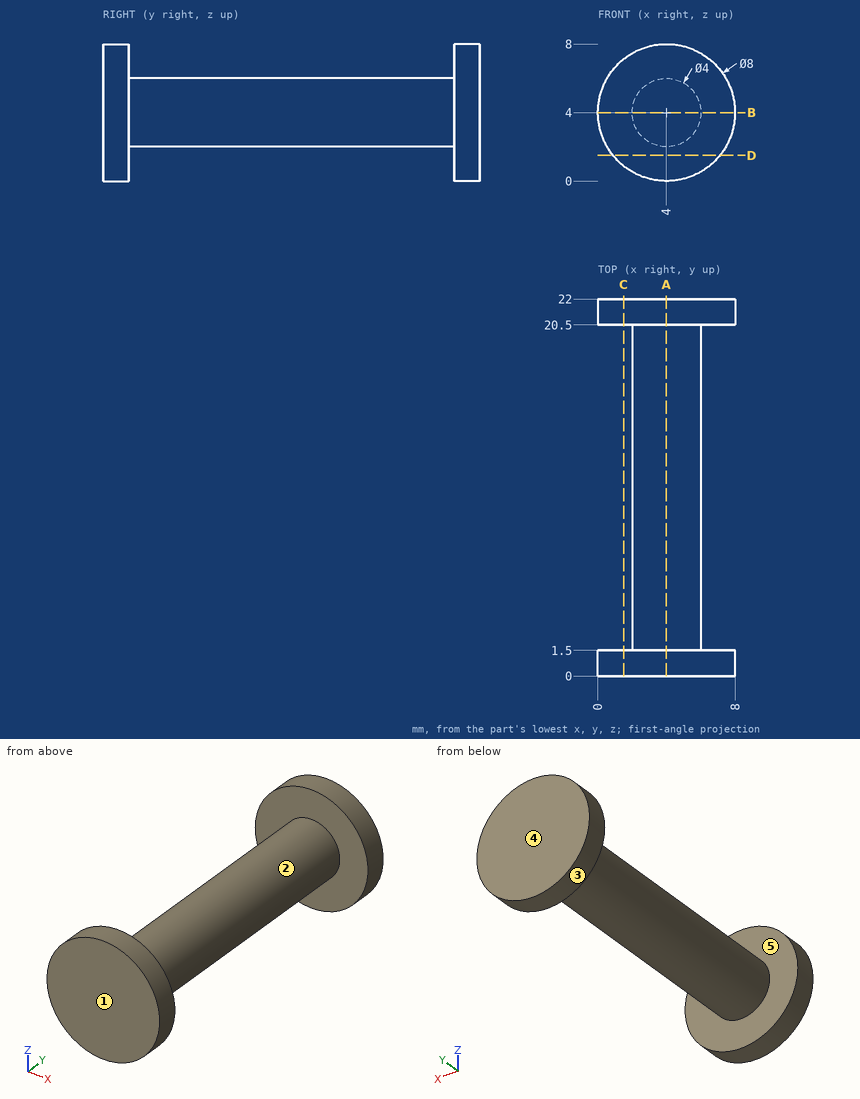
Check sheet for the drawn part. Datum: minimum x, y, z corner. Units: mm. A direction names the side the tool comes from. Round coordinates to 2 decimals unless told otherwise and drop trailing zeros. Write each loop counter-clockwise with the first axis right and the second up, starting at its lowest first coordinate (ties: lowest second). Pieces come first, ordered by that corner, then holes. Notation, with made-up numbers: (-34.75, 11) - (-9.75, 11) arc R27 ccw to (-9.75, 42) - close; hole circle Ø11 at (75, -3.75). An arc over 180 degrees is marked (long way). Return JSON: item names as keys, results as strings.
Q1. Access from +Z, -Z, +X, -X, +Y, -Y to the whole of each face (thin tool, end or side, straight path). Record for the marked faces 4 and 5.
Returned:
{"face 4": "+Z, -Z, +X, -X, +Y", "face 5": "none"}
Q2. Depth check by flat-ended pin: P1, Ø4, axis at y = 10, z = 6, coming from the -X side; P2, Ø1.5, axis at x = 1, y = 19.5, coming from the -Z side; P3, Ø4, axis at x = 6.5, y = 14.5, coming from the +Z side. Enter the tip coordinate at first touch or a pass-through.
Returned:
{"P1": "stops at x = 2", "P2": "passes through", "P3": "stops at z = 5.94"}
Q3. Scan lines: L1, parallel to Y at x = 1.5, z = 2.5; L2, parallel to Z at x = 2.5, y = 12.75; L3, parallel to Z at x = 4.75, y = 15.25. Record each from-to range of solid material in increasing order. Write a range as from..to.
Returned:
{"L1": "y = 0..1.5, 20.5..22", "L2": "z = 2.68..5.32", "L3": "z = 2.15..5.85"}
Q4. Cross-section at A-A (x = 4). Record the boundary of the cut face in (y, z), then the cut area to 3 significant figures.
Returned:
{"outline": "(0, 0) - (1.5, 0) - (1.5, 2) - (20.5, 2) - (20.5, 0) - (22, 0) - (22, 8) - (20.5, 8) - (20.5, 6) - (1.5, 6) - (1.5, 8) - (0, 8) - close", "area": "100 mm²"}
Q5. Cross-section at B-B (z = 4). Record the boundary of the cut face in (x, y), then the cut area to 3 significant figures.
Returned:
{"outline": "(0, 0) - (8, 0) - (8, 1.5) - (6, 1.5) - (6, 20.5) - (8, 20.5) - (8, 22) - (0, 22) - (0, 20.5) - (2, 20.5) - (2, 1.5) - (0, 1.5) - close", "area": "100 mm²"}
Q6. Cross-section at D-D (z = 1.5). Record the boundary of the cut face in (x, y), then the cut area to 3 significant figures.
Returned:
{"outline": "(0.88, 0) - (7.12, 0) - (7.12, 1.5) - (0.88, 1.5) - close; (0.88, 20.5) - (7.12, 20.5) - (7.12, 22) - (0.88, 22) - close", "area": "18.7 mm²"}
Q7. Draft check along Y on the marked faces 1, 2 and 3. Enter one of: released by +Y, released by -Y, zero draft, split by the parting line, or undercut.
Returned:
{"face 1": "released by -Y", "face 2": "undercut", "face 3": "zero draft"}
Q8. Cross-section at C-C (x = 1.5). Record the boundary of the cut face in (y, z).
Returned:
{"outline": "(0, 0.88) - (1.5, 0.88) - (1.5, 7.12) - (0, 7.12) - close; (20.5, 0.88) - (22, 0.88) - (22, 7.12) - (20.5, 7.12) - close"}
